```python
from build123d import *

# Parameters (mm, degrees)
SKETCH1_R           = 1.5
BOSS_EXTRUDE1_DEPTH = 4
CUT_EXTRUDE1_DEPTH  = 23.415528994
CIRPATTERN1_COUNT   = 12
SKETCH3_W           = 11.336678395
SKETCH3_H           = 5
BOSS_EXTRUDE2_DEPTH = 4
SKETCH4_R           = 2.5
CUT_EXTRUDE2_DEPTH  = 23.170725743


with BuildPart() as part:
    # Sketch1 → Boss-Extrude1 (new body)
    with BuildSketch(Plane.XY):
        with BuildLine():
            Line((-18, 2.5), (9.769591268, 2.5))
            ThreePointArc((9.769591268, 2.5), (21.223947325, 0), (9.769591268, -2.5))
            Line((9.769591268, -2.5), (-18, -2.5))
            ThreePointArc((-18, -2.5), (-20.5, 0), (-18, 2.5))
        make_face()
        with Locations((-18, 0)):
            Circle(SKETCH1_R, mode=Mode.SUBTRACT)
    extrude(amount=BOSS_EXTRUDE1_DEPTH)

    # Sketch2 → Cut-Extrude1 (cut, through all)
    with BuildSketch(Plane.XY.offset(4)):
        with BuildLine():
            Line((17.107572926, 4.746445804), (16.983821507, 4.529223369))
            ThreePointArc((16.983821507, 4.529223369), (16.945677893, 4.005263167), (17.328947325, 3.64596695))
            ThreePointArc((17.328947325, 3.64596695), (17.831741692, 3.493693994), (18.266432731, 3.788707433))
            Line((18.266432731, 3.788707433), (18.392677169, 4.004490523))
            ThreePointArc((18.392677169, 4.004490523), (18.877651327, 4.357969149), (19.466588012, 4.242640687))
            ThreePointArc((19.466588012, 4.242640687), (18.501167967, 5.676312659), (16.776861596, 5.795554958))
            ThreePointArc((16.776861596, 5.795554958), (17.171207316, 5.343185058), (17.107572926, 4.746445804))
        make_face()
    cut_extrude1 = extrude(amount=-CUT_EXTRUDE1_DEPTH, mode=Mode.SUBTRACT)

    # CirPattern1: Cut-Extrude1 ×12 about axis
    cirpattern1_axis = Axis((15.223947325, 0, 0), (0, 0, 1))
    for i in range(1, CIRPATTERN1_COUNT):
        add(cut_extrude1.rotate(cirpattern1_axis, i * 360 / CIRPATTERN1_COUNT), mode=Mode.SUBTRACT)

    # Sketch3 → Boss-Extrude2 (add)
    with BuildSketch(Plane.XY.offset(4)):
        with Locations((11.656973093, 0)):
            Rectangle(SKETCH3_W, SKETCH3_H)
    extrude(amount=-BOSS_EXTRUDE2_DEPTH)

    # Sketch4 → Cut-Extrude2 (cut, through all)
    with BuildSketch(Plane.XY.offset(4)):
        with Locations((15.223947325, 0)):
            Circle(SKETCH4_R)
    extrude(amount=-CUT_EXTRUDE2_DEPTH, mode=Mode.SUBTRACT)


solid = part.part
```
Source: CAD feature listing. Evaluate the final solid. Frame: model axes, mm. A direction names the side the tool comes from. Round coordinates to 2 decimals unless told otherwise and drop trailing zeros. Loops run counter-clockwise (first coordinate to the right, second up) from the corner with the lowest first, then second, coordinate; pieces in that order, holes last.
(1) Material intervals for probe 1 along Y at (x, z) = (-18, 0.95); probe 2 along X at (y, z) = (-0.25, 3.6); probe 3 along Y at (x, z) = (11, 1.65), sorted ascending.
From the geometry:
probe 1: y = -2.5 to -1.5, 1.5 to 2.5
probe 2: x = -20.49 to -19.48, -16.52 to 12.74, 17.71 to 19.43
probe 3: y = -4.26 to -3.36, -2.5 to 2.5, 3.36 to 4.26
(2) Contact query for flat-ended pins moving along their axis: pin 1 Ø1 at (x, z) = (-6.5, 3) entering from +Y; pin 2 Ø1.5 at (x, z) = (0, 2.5) entering from -Y; pin 3 Ø1.5 at (y, z) = (4, 1.5) entering from +X. Output: stop coordinate, or through.
From the geometry:
pin 1: stops at y = 2.5
pin 2: stops at y = -2.5
pin 3: stops at x = 19.6
(3) Pull-direction query (Y, two-part tool) for faces 1 (the cylindrical face through (18.72, 2.62, 2.03)), 2 (the flat face through (5, 0, 0)), 3 (the cylindrical face through (20.575, -1.945, 2.028)); classes: +Y half, -Y half, draft (parallel to the pull), parting line (faces both ways), or undercut.
From the geometry:
face 1: undercut
face 2: draft
face 3: -Y half
(4) Section query A-A (x = -4). Output: boundary loops of the cut face in (y, z).
From the geometry:
outline: (-2.5, 0) - (2.5, 0) - (2.5, 4) - (-2.5, 4) - close
(5) Section query B-B (z = 3.2). Give the number of separate pieces and of enclosed holes in the cut face, and give its area (3 significant figures).
From the geometry:
separate pieces: 1
enclosed holes: 2
area: 204 mm2
(6) Access query for faces 4 (the cylindrical face through (20.82, -0.98, 2.03)), 5 (the cylindrical face through (17.824, 3.493, 2.028)), 6 (the cylindrical face through (16.943, 4.012, 2.028)). Directions: +Z, -Z, +X, -X, +Y, -Y. A direction counts if a zero-diameter tool reaches every point of the face in a straight line with its end or side. Return the directions, or none.
From the geometry:
face 4: +Z, -Z, +X
face 5: +Z, -Z, +Y
face 6: +Z, -Z
